The listing builds one solid part. Answer for the finished solid, in the listing's coordinates (mm). Face numbers are marked on the shaded views. A direction names the side the tool comes from. Round coordinates to 2 decimals unless told otherwise and drop trailing zeros. Loops run counter-clockwise (first coordinate to the right, second up) from the corner with the lowest first, then second, coordinate; pieces in that order, holes last. Notation, with made-up numbers: (-17, 22) -> (36, 22) arc R21 cw to (36, 50) -> close; hole circle Ø1 at (67.25, 23.25). An arc over 180 degrees is marked (long way). Use a Markdown table: item, result. Add a question column.
Q1. Section A-A on x = -23 is taken. Give the vertices of the cut face in (y, z), then the cut area to 3 significant figures.
Q2. Section C-C on z = 20 is taken. Give the vertices of the cut face in (x, y) (3 decimals).
Q3. Which of the six approach directions +Z, -Z, +X, -X, +Y, -Y give full straight-line access (tool end or side, diameter ignored) to the marked faces 4, 5, 6, 7 and 8?
Q4. For a pull along Y with two mould halves and no side action, classify the marked faces 1, 2 and 3 as released by +Y, released by -Y, zero draft, split by the parting line, or undercut.
Q5. Section D-D on x = 0 is taken. Give the vertices of the cut face in (y, z) (3 decimals), then the cut area to 3 significant figures.
Q6. Consider line 1 (Y direction, x = 0, z = 17.3); line 2 (Z direction, x = -12.5, y = 9.5); line 3 (X direction, y = 4, z = 14.5). Determine where each line is inside the solid, lowest interval first.
Q7. Section B-B on y = 0 is taken. Give the vertices of the cut face in (x, z) (3 decimals).
Q8. Given pin 1 Ø10 at (y, z) = (7, 14) entering from -X; pin 2 Ø10 at (x, y) = (17.5, -12) entering from +Z; pin 3 Ø2 at (y, z) = (-2, 5.5) entering from -X, each flat-ended and moving along its own axis, determine where each tip first touches the part or whether it passes through.
from build123d import *

# Parameters (mm, degrees)
F0_W     = 38.1
F0_H     = 12.7
F1_DEPTH = 19.05
F2_R     = 12.7
F2_R_2   = 9.525
F3_DEPTH = 7.62
F4_R     = 1.905
F5_DEPTH = 2.54
F6_R     = 2.54


with BuildPart() as f1:
    # F0 (on Front) → F1 (new body, symmetric)
    with BuildSketch(Plane.XZ):
        Polygon((-19.05, 6.35), (-31.75, 6.35), (-31.75, -6.35), (31.75, -6.35), (31.75, 6.35), (19.05, 6.35), align=None)
        with Locations((0, 12.7)):
            Rectangle(F0_W, F0_H)
    extrude(amount=F1_DEPTH, both=True)

    # F2 (on face) → F3 (join)
    with BuildSketch(Plane.XY.offset(19.05)):
        Circle(F2_R)
        Circle(F2_R_2, mode=Mode.SUBTRACT)
    extrude(amount=F3_DEPTH)

    # F4 (on face) → F5 (cut)
    with BuildSketch(Plane.XY.offset(19.05)):
        with Locations((13.748153, -7.9375)):
            Circle(F4_R)
        with Locations((13.748153, 7.9375)):
            Circle(F4_R)
        with Locations((0, 15.875)):
            Circle(F4_R)
        with Locations((-13.748153, 7.9375)):
            Circle(F4_R)
        with Locations((-13.748153, -7.9375)):
            Circle(F4_R)
        with Locations((0, -15.875)):
            Circle(F4_R)
    extrude(amount=-F5_DEPTH, mode=Mode.SUBTRACT)

    # F6
    f6_edges = [f1.edges().sort_by_distance(p)[0] for p in [
        (25.4, 19.05, 6.35),
        (31.75, 0, 6.35),
        (25.4, -19.05, 6.35),
        (-19.05, 19.05, 12.7),
        (-25.4, 19.05, 6.35),
        (-31.75, 0, 6.35),
        (-25.4, -19.05, 6.35),
        (-19.05, -19.05, 12.7),
        (19.05, -19.05, 12.7),
        (19.05, 19.05, 12.7),
    ]]
    fillet(f6_edges, radius=F6_R)


solid = f1.part
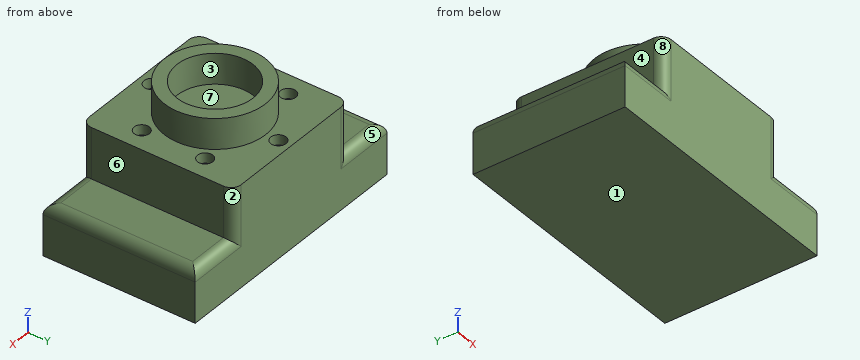
Checked values:
| question | item | result |
|---|---|---|
| 1 | outline | (-19.05, -6.35) -> (19.05, -6.35) -> (19.05, 3.81) arc R2.54 ccw to (16.51, 6.35) -> (-16.51, 6.35) arc R2.54 ccw to (-19.05, 3.81) -> close |
| 1 | area | 481 mm2 |
| 2 | outline | circle Ø25.4 at (0, 0); hole circle Ø19.05 at (0, 0) |
| 3 | face 4 | +Z, -X, +Y, -Y |
| 3 | face 5 | +Z, -X, +Y |
| 3 | face 6 | +Z, +X, +Y, -Y |
| 3 | face 7 | +Z |
| 3 | face 8 | +Z, -X, -Y |
| 4 | face 1 | zero draft |
| 4 | face 2 | released by +Y |
| 4 | face 3 | undercut |
| 5 | outline | (-19.05, -6.35) -> (19.05, -6.35) -> (19.05, 19.05) -> (17.78, 19.05) -> (17.78, 16.51) -> (13.97, 16.51) -> (13.97, 19.05) -> (12.7, 19.05) -> (12.7, 26.67) -> (9.525, 26.67) -> (9.525, 19.05) -> (-9.525, 19.05) -> (-9.525, 26.67) -> (-12.7, 26.67) -> (-12.7, 19.05) -> (-13.97, 19.05) -> (-13.97, 16.51) -> (-17.78, 16.51) -> (-17.78, 19.05) -> (-19.05, 19.05) -> close |
| 5 | area | 997 mm2 |
| 6 | line 1 | y = -19.05 to -17.78, -13.97 to 13.97, 17.78 to 19.05 |
| 6 | line 2 | z = -6.35 to 19.05 |
| 6 | line 3 | x = -19.05 to 19.05 |
| 7 | outline | (-31.75, -6.35) -> (31.75, -6.35) -> (31.75, 3.81) arc R2.54 ccw to (29.21, 6.35) -> (19.05, 6.35) -> (19.05, 19.05) -> (12.7, 19.05) -> (12.7, 26.67) -> (9.525, 26.67) -> (9.525, 19.05) -> (-9.525, 19.05) -> (-9.525, 26.67) -> (-12.7, 26.67) -> (-12.7, 19.05) -> (-19.05, 19.05) -> (-19.05, 6.35) -> (-29.21, 6.35) arc R2.54 ccw to (-31.75, 3.81) -> close |
| 8 | pin 1 | stops at x = -19.05 |
| 8 | pin 2 | stops at z = 19.05 |
| 8 | pin 3 | stops at x = -31.65 |
